Autodesk Inventor part; units mm, degrees
ref_plane "YZ Plane" through (0, 0, 0) normal (1, 0, 0) x (0, 1, 0)
ref_plane "XZ Plane" through (0, 0, 0) normal (0, 1, 0) x (-1, 0, 0)
ref_plane "XY Plane" through (0, 0, 0) normal (0, 0, 1) x (1, 0, 0)
sketch "Sketch1" plane through (0, 0, 0) normal (0, 1, 0) x (-1, 0, 0)
  line L0 (3.2881, 3.6219) -> (-4.4081, 3.6219)
  line L1 (-4.4081, 3.6219) -> (-4.4081, -2.7281)
  line L2 (-4.4081, -2.7281) -> (3.2881, -2.7281)
  line L3 (3.2881, -2.7281) -> (3.2881, 3.6219)
  point P0 (0, 0)
  dimension "d0" = 7.6962
  dimension "d1" = 6.35
extrude "Extrusion1" add sketch "Sketch1" along normal blind 2.54
sketch "Sketch2" plane through (0, 2.54, 0) normal (0, 1, 0) x (1, 0, 0)
  circle A0 centre (0.56, -0.4469) radius 1.5
  line L0 (4.4081, 2.7281) -> (-3.2881, 2.7281)
  line L1 (-3.2881, 2.7281) -> (-3.2881, -3.6219)
  point P0 (0, 0)
  point P1 (0.56, 2.7281)
  point P2 (-3.2881, -0.4469)
  dimension "d4" = 3
extrude "Extrusion2" add sketch "Sketch2" along normal blind 5.08
sketch "Sketch3" plane through (0, 0, 0) normal (0, -1, 0) x (1, 0, 0)
  line L0 (-3.2881, -2.7281) -> (-3.2881, 3.6219)
  line L1 (-3.2881, -2.7281) -> (-0.7481, -2.7281)
  line L2 (-0.7481, -2.7281) -> (-0.7481, 3.6219)
  line L3 (-0.7481, 3.6219) -> (-3.2881, 3.6219)
  line L4 (-3.2881, 3.6219) -> (-3.2881, -2.7281)
  line L5 (4.4081, -2.7281) -> (1.8681, -2.7281)
  line L6 (1.8681, -2.7281) -> (1.8681, 3.6219)
  line L7 (1.8681, 3.6219) -> (4.4081, 3.6219)
  line L8 (4.4081, 3.6219) -> (4.4081, -2.7281)
  point P0 (0, 0)
  dimension "d7" = 2.54
  dimension "d8" = 2.54
  dimension "d9" = 2.6162
extrude "Extrusion3" add sketch "Sketch3" along normal blind 20.32
equation "\"d8\" = d7"
properties part number "Control Board Ring Slot Holder"
The listing builds one solid part. Answer for the finished solid, in the listing's coordinates (mm). A direction names the side the tool comes from. Give positions to 0.01 mm unless a question says otherwise; leave off trailing zeros. Loops run counter-clockwise (first coordinate to the right, second up) from the corner with the lowest first, then second, coordinate; pieces in that order, holes last. Notation, with made-up numbers: M -22.75,30 L 29.25,30 A25 ccw 29.25,61 Z; hole C 85,28 d4. An arc over 180 degrees is marked long. Answer as CSV lines item,"result".
Item 1: Straight lines are drawn through the part: line 1 along X through (y, z) = (-17.75, -1); line 2 along Y through (x, z) = (-1, 2.5); line 3 along Z through (x, y) = (0.5, 5.5). For each, find the intervals that lie inside material, in ascending order. Write a range as [from, to].
Values follow:
line 1,"x = [-3.29, -0.75], [1.87, 4.41]"
line 2,"y = [-20.32, 2.54]"
line 3,"z = [-1.05, 1.95]"
Item 2: Which of the six approach directions +Z, -Z, +X, -X, +Y, -Y give full straight-line access (tool end or side, diameter ignored) to faces 1 (the cylindrical face through (0.235, 5.044, -1.017)), 2 (the flat face through (-1, -9, 3.622)), 3 (the flat face through (-0.748, -10, 0))?
Values follow:
face 1,"+Y"
face 2,"+Z, +X, -X, +Y, -Y"
face 3,"+Z, -Z, -Y"
Item 3: The mould has two halves that part along X. Classify faces 4 (the flat face through (1.5, 2.54, 1.9)), 5 (the flat face through (4.408, -9, 0)), 6 (the flat face through (1, 0, 0)): released by +X, released by -X, zero draft, split by the parting line, or undercut.
Values follow:
face 4,"zero draft"
face 5,"released by +X"
face 6,"undercut"
Item 4: The part is cut by section A-A (z = 3.25). Give the vertices of the cut face in (x, y).
Values follow:
outline,"M -3.29,-20.32 L -0.75,-20.32 L -0.75,0 L 1.87,0 L 1.87,-20.32 L 4.41,-20.32 L 4.41,2.54 L -3.29,2.54 Z"
Item 5: The part is cut by section B-B (x = 0.56). Give the vertices of the cut face in (y, z).
Values follow:
outline,"M 0,-2.73 L 2.54,-2.73 L 2.54,-1.05 L 7.62,-1.05 L 7.62,1.95 L 2.54,1.95 L 2.54,3.62 L 0,3.62 Z"
Item 6: Given pin 1 Ø1.3 at (x, z) = (0.5, 2) entering from -Y; pin 2 Ø2 at (x, z) = (-0.5, -2) entering from -Y, each flat-ended and moving along its own axis, determine where each tip first touches the part or whether it passes through.
Values follow:
pin 1,"stops at y = 0"
pin 2,"stops at y = -20.32"
Item 7: The part is cut by section C-C (x = -1.25). Give the vertices of the cut face in (y, z).
Values follow:
outline,"M -20.32,-2.73 L 2.54,-2.73 L 2.54,3.62 L -20.32,3.62 Z"
